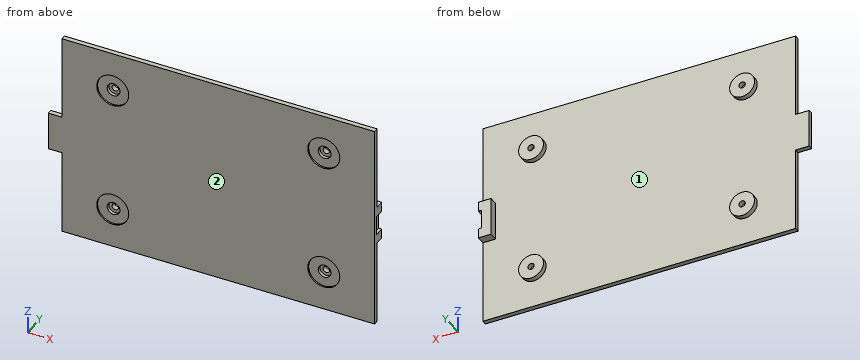
```python
from build123d import *

# Parameters (mm, degrees)
EXTRUDE_1_DEPTH     = 1.5
SKETCH_2_R          = 5
CUT_EXTRUDE_1_DEPTH = 0.5
LED_3_START         = -4.25
LED_3_DEPTH         = 2.75
CUT_EXTRUDE_2_REACH = 76.153
SKETCH_15_R         = 2
EXTRUDE_START       = -3.1
SKETCH_16_R         = 3.9
SKETCH_16_R_2       = 1
EXTRUDE_4_DEPTH     = 1.6
LED_2_START         = -1.5
SKETCH_17_W         = 1
SKETCH_17_H         = 6
LED_2_DEPTH         = 0.5


with BuildPart() as part:
    # 草图1 → 凸台-拉伸1 (new body)
    with BuildSketch(Plane(origin=(0, 0, 0), x_dir=(1, 0, 0), z_dir=(0, 1, 0))):
        Polygon((-51.714401711, -10.060969859), (-55.976720774, -10.060969859), (-55.976720774, -22.035569809), (-51.714401711, -22.035569809), (-51.714401711, -48.448269834), (46.085598289, -48.448269834), (46.085598289, 16.351730166), (-51.714401711, 16.351730166), align=None)
    extrude(amount=EXTRUDE_1_DEPTH)

    # 草图2 → 防滑切除-拉伸1 (cut)
    with BuildSketch(Plane.XZ):
        with Locations(Location((-35.814401712, 36.048269834, 0), (0, 0, 270))):
            Circle(SKETCH_2_R)
        with Locations(Location((30.185598288, -3.951730166, 0), (0, 0, 90))):
            Circle(SKETCH_2_R)
        with Locations(Location((-35.814401712, -3.951730166, 0), (0, 0, 270))):
            Circle(SKETCH_2_R)
        with Locations(Location((30.185598288, 36.048269834, 0), (0, 0, 270))):
            Circle(SKETCH_2_R)
    extrude(amount=-CUT_EXTRUDE_1_DEPTH, mode=Mode.SUBTRACT)

    # 草图14 → LED限位凸台-拉伸3 (add)
    with BuildSketch(Plane.XZ.offset(LED_3_START)):
        Polygon((45.085598289, 13.048269834), (45.085598289, 19.048269834), (46.085598289, 19.048269834), (46.085598289, 22.048269834), (42.085598289, 22.048269834), (42.085598289, 10.048269834), (46.085598289, 10.048269834), (46.085598289, 13.048269834), align=None)
    extrude(amount=LED_3_DEPTH)

    # 草图15 → 螺丝孔位切除-拉伸2 (cut, up to next)
    with BuildSketch(Plane.XZ, mode=Mode.PRIVATE) as cut_extrude_2_sk1:
        with Locations(Location((-35.814401712, 36.048269834, 0), (0, 0, 270))):
            Circle(SKETCH_15_R)
    cut_extrude_2_tool1 = extrude(cut_extrude_2_sk1.sketch, amount=-CUT_EXTRUDE_2_REACH, mode=Mode.PRIVATE) & part.part
    # 草图15 → 螺丝孔位切除-拉伸2 (cut, up to next)
    with BuildSketch(Plane.XZ, mode=Mode.PRIVATE) as cut_extrude_2_sk2:
        with Locations(Location((30.185598288, 36.048269834, 0), (0, 0, 270))):
            Circle(SKETCH_15_R)
    cut_extrude_2_tool2 = extrude(cut_extrude_2_sk2.sketch, amount=-CUT_EXTRUDE_2_REACH, mode=Mode.PRIVATE) & part.part
    # 草图15 → 螺丝孔位切除-拉伸2 (cut, up to next)
    with BuildSketch(Plane.XZ, mode=Mode.PRIVATE) as cut_extrude_2_sk3:
        with Locations(Location((30.185598288, -3.951730166, 0), (0, 0, 90))):
            Circle(SKETCH_15_R)
    cut_extrude_2_tool3 = extrude(cut_extrude_2_sk3.sketch, amount=-CUT_EXTRUDE_2_REACH, mode=Mode.PRIVATE) & part.part
    # 草图15 → 螺丝孔位切除-拉伸2 (cut, up to next)
    with BuildSketch(Plane.XZ, mode=Mode.PRIVATE) as cut_extrude_2_sk4:
        with Locations(Location((-35.814401712, -3.951730166, 0), (0, 0, 270))):
            Circle(SKETCH_15_R)
    cut_extrude_2_tool4 = extrude(cut_extrude_2_sk4.sketch, amount=-CUT_EXTRUDE_2_REACH, mode=Mode.PRIVATE) & part.part
    add(cut_extrude_2_tool1.solids().sort_by_distance((-35.814402, 0, 36.04827))[0], mode=Mode.SUBTRACT)
    add(cut_extrude_2_tool2.solids().sort_by_distance((30.185598, 0, 36.04827))[0], mode=Mode.SUBTRACT)
    add(cut_extrude_2_tool3.solids().sort_by_distance((30.185598, 0, -3.95173))[0], mode=Mode.SUBTRACT)
    add(cut_extrude_2_tool4.solids().sort_by_distance((-35.814402, 0, -3.95173))[0], mode=Mode.SUBTRACT)

    # 草图16 → 螺丝孔凸台-拉伸4 (add)
    # profile 1 of 4: a face of its own
    with BuildSketch(Plane.XZ.offset(EXTRUDE_START)):
        with Locations(Location((-35.814401712, 36.048269834, 0), (0, 0, 180))):
            Circle(SKETCH_16_R)
        with Locations(Location((-35.814401712, 36.048269834, 0), (0, 0, 180))):
            Circle(SKETCH_16_R_2, mode=Mode.SUBTRACT)
    # profile 2 of 4: a face of its own
    with BuildSketch(Plane.XZ.offset(EXTRUDE_START)):
        with Locations(Location((30.185598288, 36.048269834, 0), (0, 0, 180))):
            Circle(SKETCH_16_R)
        with Locations(Location((30.185598288, 36.048269834, 0), (0, 0, 180))):
            Circle(SKETCH_16_R_2, mode=Mode.SUBTRACT)
    # profile 3 of 4: a face of its own
    with BuildSketch(Plane.XZ.offset(EXTRUDE_START)):
        with Locations(Location((30.185598288, -3.951730166, 0), (0, 0, 180))):
            Circle(SKETCH_16_R)
        with Locations(Location((30.185598288, -3.951730166, 0), (0, 0, 180))):
            Circle(SKETCH_16_R_2, mode=Mode.SUBTRACT)
    # profile 4 of 4: a face of its own
    with BuildSketch(Plane.XZ.offset(EXTRUDE_START)):
        with Locations(Location((-35.814401712, -3.951730166, 0), (0, 0, 180))):
            Circle(SKETCH_16_R)
        with Locations(Location((-35.814401712, -3.951730166, 0), (0, 0, 180))):
            Circle(SKETCH_16_R_2, mode=Mode.SUBTRACT)
    extrude(amount=EXTRUDE_4_DEPTH)

    # 草图17 → LED灯嵌入切除-拉伸2 (cut)
    with BuildSketch(Plane.XZ.offset(LED_2_START)):
        with Locations((45.585598289, 16.048269834)):
            Rectangle(SKETCH_17_W, SKETCH_17_H)
    extrude(amount=LED_2_DEPTH, mode=Mode.SUBTRACT)


solid = part.part
```
Input: part model. Units: mm. Frame: model coordinates. Face numbers are marked on the shaded views. Give positions to 0.01 mm unless a question says otherwise; leave off trailing zeros. Order: outer loops, then holes, each group sorted by start corner. A loop starts at its lowest first (then second) coordinate and runs counter-clockwise, first axis right, second up. Notation, with made-up numbers: M 49.5,58.5 L 89.5,58.5 A10 ccw 89.5,77.5 Z; hole C -30,40.5 d6. An arc over 180 degrees is marked long. Return JSON: item names as keys, results as strings.
Item 1: Pull-direction query (X, two-part tool) for the marked faces 1 and 2; classes: +X half, -X half, draft (parallel to the pull), parting line (faces both ways), or undercut.
Solutions:
{"face 1": "undercut", "face 2": "draft"}
Item 2: Ray query, probe 1 along Z at (x, y) = (-34, 0.2); probe 2 along Y at (x, z) = (37, 5); probe 3 along X at (y, z) = (1.15, 5). Return the intervals inside material, ascending.
Solutions:
{"probe 1": "-16.35 to -8.61, 0.71 to 31.39, 40.71 to 48.45", "probe 2": "0 to 1.5", "probe 3": "-51.71 to 46.09"}
Item 3: First-contact query: P1, Ø1.6, axis at y = 0.5, z = -0.5, coming from the -X side; P2, Ø3, axis at x = 30.19, z = -3.95, coming from the -Y side; P3, Ø2.5, axis at x = 30.19, z = -3.95, coming from the +Y side. Flat tips, straight axial feed; report the tip coordinate or a pass-through.
Solutions:
{"P1": "x = -51.71", "P2": "y = 1.5", "P3": "y = 3.1"}
Item 4: Cut plane B-B (z = -11). Return loops of the section in (x, y).
Solutions:
{"outline": "M -51.71,0 L 46.09,0 L 46.09,1.5 L -51.71,1.5 Z"}
Item 5: Cut plane A-A (x = -7). Return loops of the section in (y, z).
Solutions:
{"outline": "M 0,-16.35 L 1.5,-16.35 L 1.5,48.45 L 0,48.45 Z"}
